Design review of the part built by this model. Coordinates are the model's own, in mm. Face numbers are marked on the shaded views. A direction names the side the tool comes from. Coordinates: 2 decimals unless noted, no trailing zeros. Loops run counter-clockwise (first coordinate to the right, second up) from the corner with the lowest first, then second, coordinate; pieces in that order, holes last. Notation, with made-up numbers: M -5.75,44 L 34.25,44 A5 ccw 34.25,50 Z; hole C 42,82 d9. An arc over 180 degrees is marked long. Answer as a JSON object with one key per item and string values. Group by question number.
1. Machinability: for the marked faces 5, 6, 7, 8 and 9, which of the approach directions +Z, -Z, +X, -X, +Y, -Y give a long, thin tool a straight path to every point of the face, cutting with its end or side? Answer none if there is none.
2. To check wall thickness, follow probe 1 along Z at (x, y) = (15.75, 6); probe 2 along Z at (x, y) = (-7, 5.25); probe 3 along Y at (x, z) = (13, -2.3). State the ranges of each line that lie inside material, in increasing order.
3. Consider section B-B (x = -9). State the section outline as (y, z) points.
4. Consider section C-C (x = 13). State the section outline as (y, z) points.
5. Consider section D-D (z = 6). State the section outline as (x, y) points, then the cut area to 3 significant figures.
6. Consider section A-A (y = 4). State the section outline as (x, z) points, then the cut area to 3 significant figures.
7. Draft analysis for pull direction X (two halves, no side actions). For the marked faces 1, 2, 3 and 4, state which applies: +X half, -X half, draft (parallel to the pull), parting line (faces both ways), or undercut.
8. Insertion check: pin 1 (6 mm diameter, centred on x = 4.5, z = -2, fed in from +Y); pin 2 (4 mm diameter, centred on x = 14, y = 5.5, fed in from +Z); pin 3 (4.5 mm diameter, centred on x = -8, y = 1.5, fed in from +Z); pin 4 (1.3 mm diameter, centred on x = 13, y = 4, fed in from +Z). Each pin has a flat end and moves straight along its axis. Give the tip position at first contact, or say it passes through.
Autodesk Inventor part; units mm, degrees
ref_plane "Work Plane1" through (0, 0.5, 0) normal (0, -1, 0) x (1, 0, 0)
ref_plane "YZ Plane" through (0, 0, 0) normal (1, 0, 0) x (0, 1, 0)
ref_plane "XZ Plane" through (0, 0, 0) normal (0, 1, 0) x (-1, 0, 0)
sketch "Sketch1" plane through (0, 0, 0) normal (0, 1, 0) x (-1, 0, 0)
  circle A0 centre (0, 0) radius 7.5
  circle A1 centre (0, 0) radius 10.5
  line L0 (0, 0) -> (5.6818, 8.8299) construction
  line L1 (0, 0) -> (0, 10.5)
  line L2 (6.222, 8.6714) -> (10.222, 8.6714)
  arc A2 (5.6818, 8.8299) -> (6.222, 8.6714) centre (6.222, 9.6714) ccw
  line L3 (6.222, 5.6714) -> (10.222, 5.6714)
  arc A3 (4.0584, 6.3071) -> (6.222, 5.6714) centre (6.222, 9.6714) ccw
  line L4 (10.222, 8.6714) -> (10.222, 5.6714) construction
  arc A4 (10.222, 5.6714) -> (10.222, 8.6714) centre (10.222, 7.1714) ccw
  line L5 (0, 0) -> (7.5, 0)
  line L6 (6.222, -8.6714) -> (10.222, -8.6714)
  arc A5 (6.222, -8.6714) -> (5.6818, -8.8299) centre (6.222, -9.6714) ccw
  line L7 (6.222, -5.6714) -> (10.222, -5.6714)
  arc A6 (6.222, -5.6714) -> (4.0584, -6.3071) centre (6.222, -9.6714) ccw
  arc A7 (10.222, -8.6714) -> (10.222, -5.6714) centre (10.222, -7.1714) ccw
  point P0 (4.0584, -6.3071)
  dimension "d0" = 15
  dimension "d1" = 3
  dimension "d2" = 32.76
  dimension "d3" = 1
  dimension "d4" = 3
  dimension "d5" = 4
  dimension "d6" = 6.222
  dimension "d7" = 4
extrude "Extrusion1" add sketch "Sketch1" along normal blind 6 contours A0 L1 A1 L3 A3 | A6 L7 A1 L1 A0 | A1 A2 L2 A4 L3 | L7 A7 L6 A5 A1
sketch "Sketch2" plane through (0, 0, 0) normal (0, -1, 0) x (1, 0, 0)
  arc A0 (-5.6818, -8.8299) -> (-5.6818, 8.8299) centre (0, 0) ccw
  line L0 (6.8739, 3) -> (17.234, 3)
  line L1 (17.234, 3) -> (17.234, -3)
  line L2 (17.234, -3) -> (6.8739, -3)
  line L3 (6.8739, -3) -> (6.8739, 3)
  line L4 (10.5, 0) -> (17.234, 0)
  arc A1 (-4.0584, -6.3071) -> (-4.0584, 6.3071) centre (0, 0) ccw
  circle A2 centre (0, 0) radius 7.5
  arc A3 (-5.6818, -8.8299) -> (-5.6818, 8.8299) centre (0, 0) ccw
  line L5 (10, -1.5) -> (16, -1.5)
  line L6 (16, -1.5) -> (16, 1.5)
  line L7 (16, 1.5) -> (10, 1.5)
  line L8 (10, 1.5) -> (10, -1.5)
  arc A4 (-4.0584, -6.3071) -> (-4.0584, 6.3071) centre (0, 0) ccw
  point P0 (10.0623, 3)
  point P1 (13.867, 0)
  point P2 (6.8739, -3)
  point P3 (10, 0)
  point P4 (7.5, 0)
  dimension "d11" = 6
  dimension "d12" = 1.234
  dimension "d14" = 6
  dimension "d20" = 2.5
  dimension "d25" = 3
extrude "Extrusion2" add sketch "Sketch2" against normal blind 8 contours L2 A1 L0 A0 L7 L8 L5 | A0 L5 L6 L4 L1 L2 | L5 L8 L7 A0 | A0 L4 L6 L5 | A0 L7 L6 L4 | L4 L6 L7 A0 L0 L1
ref_plane "Work Plane1" through (0, 0.5, 0) normal (0, -1, 0) x (1, 0, 0)
extrude "Extrusion3" cut sketch "Sketch2" against normal blind 8 from surface at -0.5 contours L5 L8 L7 A0 | A0 L4 L6 L5 | A0 L7 L6 L4
sketch "Sketch3" plane through (10.0623, 0, 3) normal (0, 0, 1) x (1, 0, 0)
  circle A0 centre (2.9377, 4) radius 1.05
  line L0 (5.9377, 0.5) -> (-0.0623, 0.5)
  point P0 (-10.0623, 0)
  point P1 (2.9377, 0.5)
  dimension "d21" = 2.1
  dimension "d22" = 3.5
extrude "Extrusion4" cut sketch "Sketch3" against normal through all
properties part number "sujetador_marcador_v2"
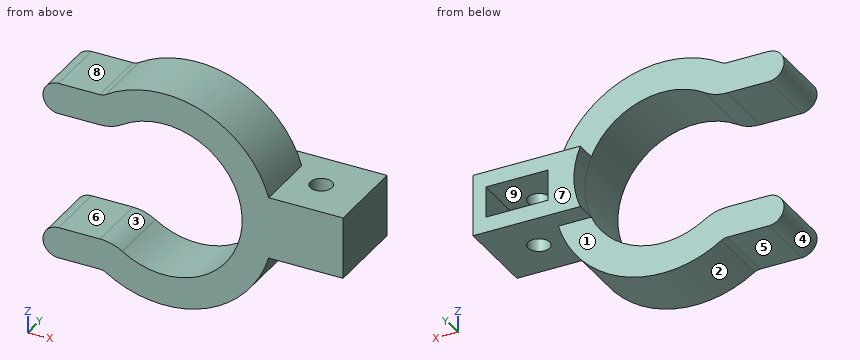
Findings below:
{
 "1": {"face 5": "-Z, -X, +Y, -Y", "face 6": "-X, +Y, -Y", "face 7": "+Z, -Z, +X, -X, +Y", "face 8": "+Z, -X, +Y, -Y", "face 9": "+Y"},
 "2": {"probe 1": "z = -3 to -1.5, 1.5 to 3", "probe 2": "z = -8.67 to -5.67, 5.67 to 8.67", "probe 3": "y = 0 to 2.95, 5.05 to 8"},
 "3": {"outline": "M 0,-8.67 L 6,-8.67 L 6,-5.67 L 0,-5.67 Z; M 0,5.67 L 6,5.67 L 6,8.67 L 0,8.67 Z"},
 "4": {"outline": "M 0,-3 L 2.95,-3 L 2.95,-1.5 L 0.5,-1.5 L 0.5,1.5 L 2.95,1.5 L 2.95,3 L 0,3 Z; M 5.05,-3 L 8,-3 L 8,-1.5 L 5.05,-1.5 Z; M 5.05,1.5 L 8,1.5 L 8,3 L 5.05,3 Z"},
 "5": {"outline": "M -11.16,0 L -4.63,0 L -4.63,6 L -11.16,6 Z; M 4.5,0 L 8.62,0 L 8.62,6 L 4.5,6 Z", "area": "63.8 mm^2"},
 "6": {"outline": "M -10.22,-8.67 L -6.22,-8.67 A1 cw -5.68,-8.83 A10.5 ccw 10.06,-3 L 11.95,-3 L 11.95,-1.5 L 10,-1.5 L 10,1.5 L 11.95,1.5 L 11.95,3 L 10.06,3 A10.5 ccw -5.68,8.83 A1 cw -6.22,8.67 L -10.22,8.67 A1.5 ccw -10.22,5.67 L -6.22,5.67 A4 ccw -4.06,6.31 A7.5 cw long -4.06,-6.31 A4 ccw -6.22,-5.67 L -10.22,-5.67 A1.5 ccw Z; M 14.05,-3 L 17.23,-3 L 17.23,3 L 14.05,3 L 14.05,1.5 L 16,1.5 L 16,-1.5 L 14.05,-1.5 Z", "area": "172 mm^2"},
 "7": {"face 1": "draft", "face 2": "parting line", "face 3": "undercut", "face 4": "-X half"},
 "8": {"pin 1": "stops at y = 8", "pin 2": "stops at z = 3", "pin 3": "stops at z = 8.79", "pin 4": "passes through"}
}
